Verification items for the finished model (mm, model axes). Face numbers are marked on the shaded views. A direction names the side the tool comes from. Coordinates: 2 decimals unless noted, no trailing zeros. Write each loop counter-clockwise with the first axis right and the second up, starting at its lowest first coordinate (ties: lowest second). Pieces come first, ordered by that corner, then holes. Notation, with made-up numbers: (-39, 67.25) - (-27, 67.25) arc R16 cw to (-27, 75.25) - close; hole circle Ø1 at (47, -16). An arc over 180 degrees is marked (long way). Use one line per item in the form item = value. Start each with the question number.
(1) Tool access check on the marked faces 5 and 6. Record the directions out of +Z, -Z, +X, -X, +Y, -Y that give a thin tool (end or side, any length) a straight path to the whole face; none if there is none.
(2) Sectioned sample at B-B (y = 8). Record the cut outline in (x, z).
(3) Mould release check, pull along Z, two halves, no side actions. Record for the marked faces 1, 2, 3 and 4: released by +Z, released by -Z, zero draft, split by the parting line, or undercut.
(4) Material ranges on line 1 (Z direction, x = 3.25, y = -7.75); line 2 (Y direction, x = 0.75, z = 12); line 3 (X direction, y = -0.5, z = 2), recorded low to high. Write a range as [from, to].
(5) Gauge pin test, flat ends, axial feed: pin 1 Ø8 at (x, y) = (6, 2) entering from +Z; pin 2 Ø4 at (y, z) = (0.5, 8.5) entering from -X; pin 3 Ø10 at (x, z) = (7, 7) entering from +Y. Record the tip position at first contact, or that the pin passes through.
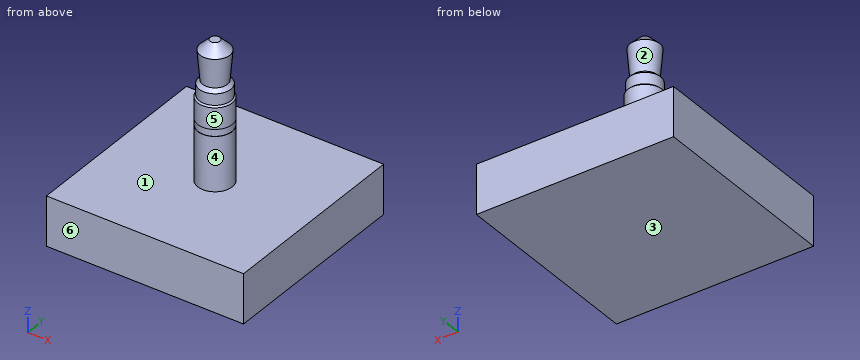
from build123d import *

# Parameters (mm, degrees)
F0_R      = 1.75
F1_DEPTH  = 5.5
F3_R      = 1.725
F4_DEPTH  = 0.7
F6_R      = 1.75
F7_DEPTH  = 2.3
F9_R      = 1.6
F10_DEPTH = 0.7
F12_R     = 1.6
F13_DEPTH = 0.8
F15_R     = 1.25
F17_R     = 1.5
F20_R     = 1.5
F21_DEPTH = 1
F22_SIZE2 = 0.99999
F22_SIZE  = 0.99999
F23_SIZE  = 0.14999
F24_SIZE  = 0.34999
F26_W     = 20
F26_H     = 20
F27_DEPTH = 5


# Not quite as in the source:
# - a fillet or chamfer is up to 0.001 mm smaller than in the source, because OpenCascade refuses the exact size


with BuildPart() as f1:
    # F0 (on Top) → F1 (new body)
    with BuildSketch(Plane.XY):
        Circle(F0_R)
    extrude(amount=F1_DEPTH)

    # F3 (on offset) → F4 (join)
    with BuildSketch(Plane.XY.offset(5.5)):
        Circle(F3_R)
    extrude(amount=F4_DEPTH)

    # F6 (on offset) → F7 (join)
    with BuildSketch(Plane.XY.offset(6.2)):
        Circle(F6_R)
    extrude(amount=F7_DEPTH)

    # F9 (on offset) → F10 (join)
    with BuildSketch(Plane.XY.offset(8.5)):
        Circle(F9_R)
    extrude(amount=F10_DEPTH)

    # F12 (on offset) → F13 (join)
    with BuildSketch(Plane.XY.offset(9.2)):
        Circle(F12_R)
    extrude(amount=F13_DEPTH)

    # F15 (on offset) → F18 section 0
    with BuildSketch(Plane.XY.offset(10)):
        Circle(F15_R)
    # F17 (on offset) → F18 section 1
    with BuildSketch(Plane.XY.offset(13)):
        Circle(F17_R)
    loft()

    # F20 (on offset) → F21 (join)
    with BuildSketch(Plane.XY.offset(13)):
        Circle(F20_R)
    extrude(amount=F21_DEPTH)

    # F22 (size 1 and 1 in the source; OpenCascade refuses exactly that, so slightly less here)
    f22_edges = [f1.edges().sort_by_distance(p)[0] for p in [
        (-1.5, 0, 14),
    ]]
    chamfer(f22_edges, length=F22_SIZE, length2=F22_SIZE2)

    # F23 (size 0.15 in the source; OpenCascade refuses exactly that, so slightly less here)
    f23_edges = [f1.edges().sort_by_distance(p)[0] for p in [
        (-1.75, 0, 8.5),
    ]]
    chamfer(f23_edges, length=F23_SIZE)

    # F24 (size 0.35 in the source; OpenCascade refuses exactly that, so slightly less here)
    f24_edges = [f1.edges().sort_by_distance(p)[0] for p in [
        (-1.6, 0, 10),
    ]]
    chamfer(f24_edges, length=F24_SIZE)

    # F26 (on offset) → F27 (join)
    with BuildSketch(Plane(origin=(0, 0, 0), x_dir=(1, 0, 0), z_dir=(0, 0, -1))):
        Rectangle(F26_W, F26_H)
    extrude(amount=F27_DEPTH)


solid = f1.part
Answers below:
q1.face_5 = +Z
q1.face_6 = +Z, -Z, +X, -X, -Y
q2.outline = (-10, -5) - (10, -5) - (10, 0) - (-10, 0) - close
q3.face_1 = released by +Z
q3.face_2 = undercut
q3.face_3 = released by -Z
q3.face_4 = zero draft
q4.line_1 = [-5, 0]
q4.line_2 = [-1.2, 1.2]
q4.line_3 = [-1.68, 1.68]
q5.pin_1 = 0
q5.pin_2 = -1.75
q5.pin_3 = through
